Geometry check sheet. Reference: the model listing, model coordinates, mm. A direction names the side the tool comes from. Give positions to 0.01 mm unless a question says otherwise; leave off trailing zeros. Order: outer loops, then holes, each group sorted by start corner. A loop starts at its lowest first (then second) coordinate and runs counter-clockwise, first axis right, second up. Notation, with made-up numbers: M 44.25,73 L 101.25,73 A18 cw 101.25,96 Z; hole C 83.25,13 d8. An arc over 180 degrees is marked long. Answer as CSV lines item,"result".
Autodesk Inventor part; units mm, degrees
ref_plane "YZ Plane" through (0, 0, 0) normal (1, 0, 0) x (0, 1, 0)
ref_plane "XZ Plane" through (0, 0, 0) normal (0, 1, 0) x (-1, 0, 0)
ref_plane "XY Plane" through (0, 0, 0) normal (0, 0, 1) x (1, 0, 0)
sketch "Boceto1" plane through (0, 0, 0) normal (0, 0, 1) x (1, 0, 0)
  circle A0 centre (0, 0) radius 7.9375
  circle A1 centre (0, 0) radius 9.4375
  dimension "d0" = 15.875
  dimension "d1" = 18.875
extrude "Extrusión1" add sketch "Boceto1" along normal mid plane 6.35
sketch "Boceto2" plane through (0, 0, 0) normal (1, 0, 0) x (0, 1, 0)
  line L0 (9.4375, 3.175) -> (12.1375, 3.175)
  line L1 (12.4375, 3.475) -> (12.4375, 4.375)
  line L2 (12.1375, 4.675) -> (9.4375, 4.675)
  arc A0 (9.4375, 4.675) -> (7.9375, 3.175) centre (9.4375, 3.175) ccw
  arc A1 (12.1375, 3.175) -> (12.4375, 3.475) centre (12.1375, 3.475) ccw
  arc A2 (12.4375, 4.375) -> (12.1375, 4.675) centre (12.1375, 4.375) ccw
  line L3 (9.4375, 3.175) -> (7.9375, 3.175)
  line L4 (0, -0.6796) -> (0, 4.0778)
  point P0 (0, 0)
  point P1 (12.4375, 3.175)
  point P2 (12.4375, 4.675)
  dimension "d4" = 3
  dimension "d5" = 1.5
  dimension "d6" = 3
  dimension "d7" = 0.3
revolve "Revolución1" add sketch "Boceto2" angle 360 about axis through (0, 0, -10) along (0, 0, 1)
properties part number "buje_carro_zona_calor"
(1) Gauge pin test, flat ends, axial feed: P1, Ø2, axis at y = -9.5, z = 1, coming from the +X side; P2, Ø3, axis at y = -7.5, z = 0, coming from the -X side; P3, Ø1.5, axis at y = 9, z = -1, coming from the -X side. Record the tip position at first contact, or that the pin passes through.
The answers:
P1,"stops at x = 4.1"
P2,"stops at x = -7.28"
P3,"stops at x = -4.58"
(2) Material ranges on line 1 (Y direction, x = 0, z = -1); line 2 (X direction, y = -6, z = -1.75), recorded low to high.
The answers:
line 1,"y = -9.44 to -7.94, 7.94 to 9.44"
line 2,"x = -7.28 to -5.2, 5.2 to 7.28"
(3) Section check D-D on z = 4. Enter the section's corners in (x, y) (1 decimal), then the cut area to 3 significant figures.
The answers:
outline,"C 0,0 d24.9; hole C 0,0 d16.4"
area,"276 mm2"
(4) Draft check along Y on faces 1 (the face through (-1.72, 7.75, -0.04)), 2 (the face through (10, 0, 3.175)), 3 (the face through (7.57, -9.87, 3.93)). Enter one of: +Y half, -Y half, draft (parallel to the pull), parting line (faces both ways), or undercut.
The answers:
face 1,"undercut"
face 2,"draft"
face 3,"parting line"
(5) Tool access check on faces 4 (the face through (9.002, -2.835, -0.044)), 5 (the face through (-2, 8, -3.175)). Record the directions out of +Z, -Z, +X, -X, +Y, -Y that give a thin tool (end or side, any length) a straight path to the whole face; none if there is none.
The answers:
face 4,"-Z"
face 5,"-Z, +X, -X, +Y, -Y"
(6) Section check C-C on z = -2.25. Enter the section's corners in (x, y) (1 decimal), then the cut area to 3 significant figures.
The answers:
outline,"C 0,0 d18.9; hole C 0,0 d15.9"
area,"81.9 mm2"
(7) Section check A-A on x = 0. Enter the section's corners in (y, z) (1 decimal), then the cut area to 3 significant figures.
The answers:
outline,"M -12.4,3.5 A0.3 ccw -12.1,3.2 L -9.4,3.2 L -9.4,-3.2 L -7.9,-3.2 L -7.9,3.2 A1.5 ccw -9.4,4.7 L -12.1,4.7 A0.3 ccw -12.4,4.4 Z; M 7.9,-3.2 L 9.4,-3.2 L 9.4,3.2 L 12.1,3.2 A0.3 ccw 12.4,3.5 L 12.4,4.4 A0.3 ccw 12.1,4.7 L 9.4,4.7 A1.5 ccw 7.9,3.2 Z"
area,"31.5 mm2"
